Job drawing, mm, ordinate dimensions from the low corner. One solid piece. A direction names the side the tool comes from. Give positions to 0.01 mm unless a question says otherwise; leave off trailing zeros. Write each loop counter-clockwise with the first axis right and the second up, starting at its lowest first coordinate (ties: lowest second). Pieces come first, ordered by that corner, then holes. Notation, with made-up numbers: (22, -27) - (52, -27) arc R34 ccw to (52, 6) - close; hole circle Ø10 at (42.5, -29). An arc over 180 degrees is marked (long way). Answer as a JSON object with one key per item and string values.
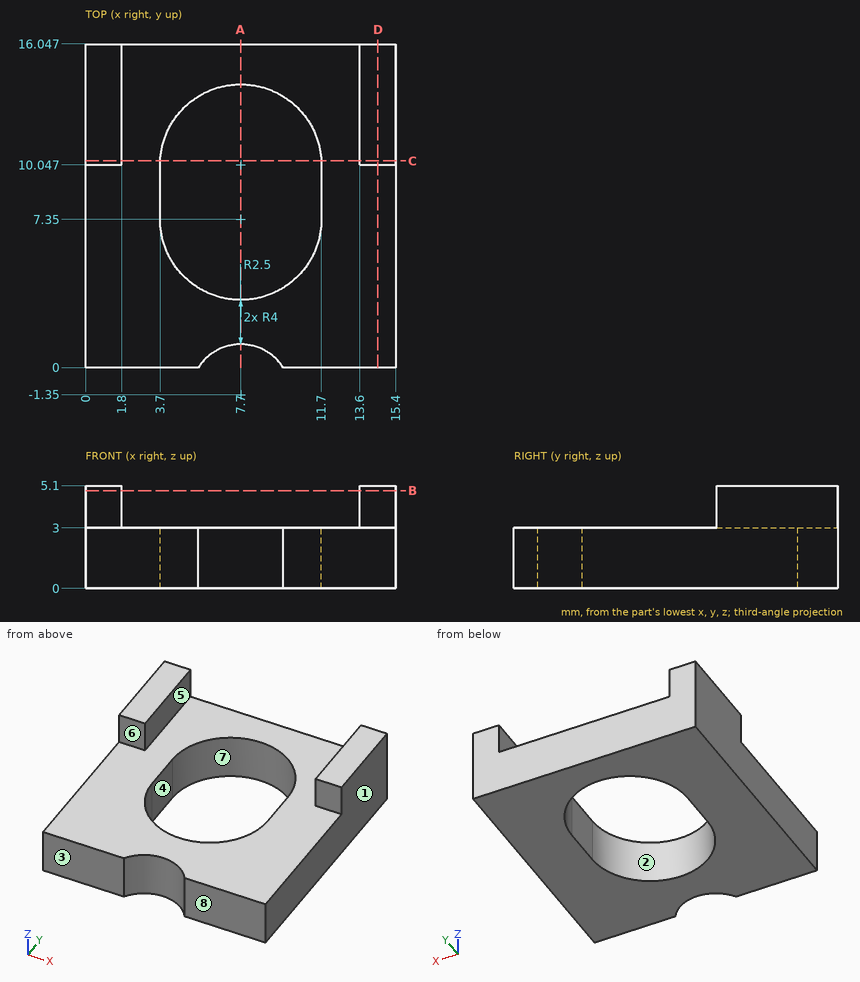
Item 1: Probe line 1 (X direction, y = 11.5, z = 3.55); line 2 (X direction, y = 7.5, z = 2.2); line 3 (Z direction, x = 12.5, y = 10.75). List the from-to ranges inside material, lowest first. Write a range as from..to.
Entries:
{"line 1": "0..1.8, 13.6..15.4", "line 2": "0..3.7, 11.7..15.4", "line 3": "0..3"}
Item 2: Flat gauge pin, fed straight in: P1, Ø3, axis at x = 2, y = 2.5, coming from the +Z side. Where does the tip first touch, or does it go through?
Entries:
{"P1": "z = 3"}
Item 3: Cut at D-D (x = 14.5). Give the cut face in (y, z).
Entries:
{"outline": "(0, 0) - (16.05, 0) - (16.05, 5.1) - (10.05, 5.1) - (10.05, 3) - (0, 3) - close"}
Item 4: Cut at B-B (z = 4.85). Give the cut face in (x, y), and give its area (3 significant figures).
Entries:
{"outline": "(0, 10.05) - (1.8, 10.05) - (1.8, 16.05) - (0, 16.05) - close; (13.6, 10.05) - (15.4, 10.05) - (15.4, 16.05) - (13.6, 16.05) - close", "area": "21.6 mm2"}
Item 5: Cut at C-C (y = 10.25). Give the cut face in (x, z) (1 decimal), and give its area (3 significant figures).
Entries:
{"outline": "(0, 0) - (3.7, 0) - (3.7, 3) - (1.8, 3) - (1.8, 5.1) - (0, 5.1) - close; (11.7, 0) - (15.4, 0) - (15.4, 5.1) - (13.6, 5.1) - (13.6, 3) - (11.7, 3) - close", "area": "29.8 mm2"}
Item 6: Which spindle directions (+Z, -Z, +X, -X, +Y, -Y) get a long thin tool onto all of the face, cutting with end or side? Do the marked faces 5, 6, 7 and 8. Say none if no direction does.
Entries:
{"face 5": "+Z, +Y, -Y", "face 6": "+Z, +X, -X, -Y", "face 7": "+Z, -Z", "face 8": "+Z, -Z, +X, -X, -Y"}
Item 7: Mould opens along Y. For the marked faces 1, 2, 3 and 4 say: +Y half, -Y half, draft (parallel to the pull), parting line (faces both ways), or undercut.
Entries:
{"face 1": "draft", "face 2": "undercut", "face 3": "-Y half", "face 4": "undercut"}
Item 8: Cut at A-A (x = 7.7). Give the cut face in (y, z).
Entries:
{"outline": "(1.15, 0) - (3.35, 0) - (3.35, 3) - (1.15, 3) - close; (14.05, 0) - (16.05, 0) - (16.05, 3) - (14.05, 3) - close"}
